Check sheet for the drawn part. Datum: minimum x, y, z corner. Units: mm. Round coordinates to 2 decimals unless told otherwise and drop trailing zeros. Write each loop counter-clockwise with the first axis right and the second up, starting at its lowest first coordinate (ties: lowest second). Pieces come first, ordered by that corner, then holes. Notation, with made-up numbers: M 64.25,-34 L 89.25,-34 A22 cw 89.25,-25 Z; hole C 45.25,4.25 d9. An arc over 180 degrees is marked long. One line per item, written item: value. Start each with the question number.
Item 1: Section check B-B, the plane y = 43. Record the cut outline in (x, z) (1 decimal), then the cut area to 3 significant figures.
Item 2: Section check D-D, the plane y = 35. Record the cut outline in (x, z), then the cut area to 3 significant figures.
Item 3: Gauge pin test, flat ends, axial feed: pin 1 (11 mm diameter, centred on x = 11, z = 38, fed in from -Y); pin 2 (6.5 mm diameter, centred on x = 17.5, z = 45, fed in from +Y); pin 3 (4 mm diameter, centred on x = 5, z = 61, fed in from -Y). Record the tip position at first contact, or that the pin passes through.
Item 4: Draft check along X on the marked faces 1, 2, 3 and 4. Enter one of: +X half, -X half, draft (parallel to the pull), parting line (faces both ways), or undercut.
Item 5: Thickness scan on probe 1 along X at (y, z) = (22.5, 23.5); probe 2 along Z at (x, y) = (11.75, 27.25); probe 3 along Y at (x, z) = (6, 45). Record the ranges inside material, lowest first. Write a range as from..to.
Item 6: Section check A-A, the plane z = 39. Record the cut outline in (x, y), then the cut area to 3 significant figures.
Item 7: Section check C-C, the plane x = 15. State how many separate pieces and enclosed holes the cut face has, then the cut area to 4 significant figures.
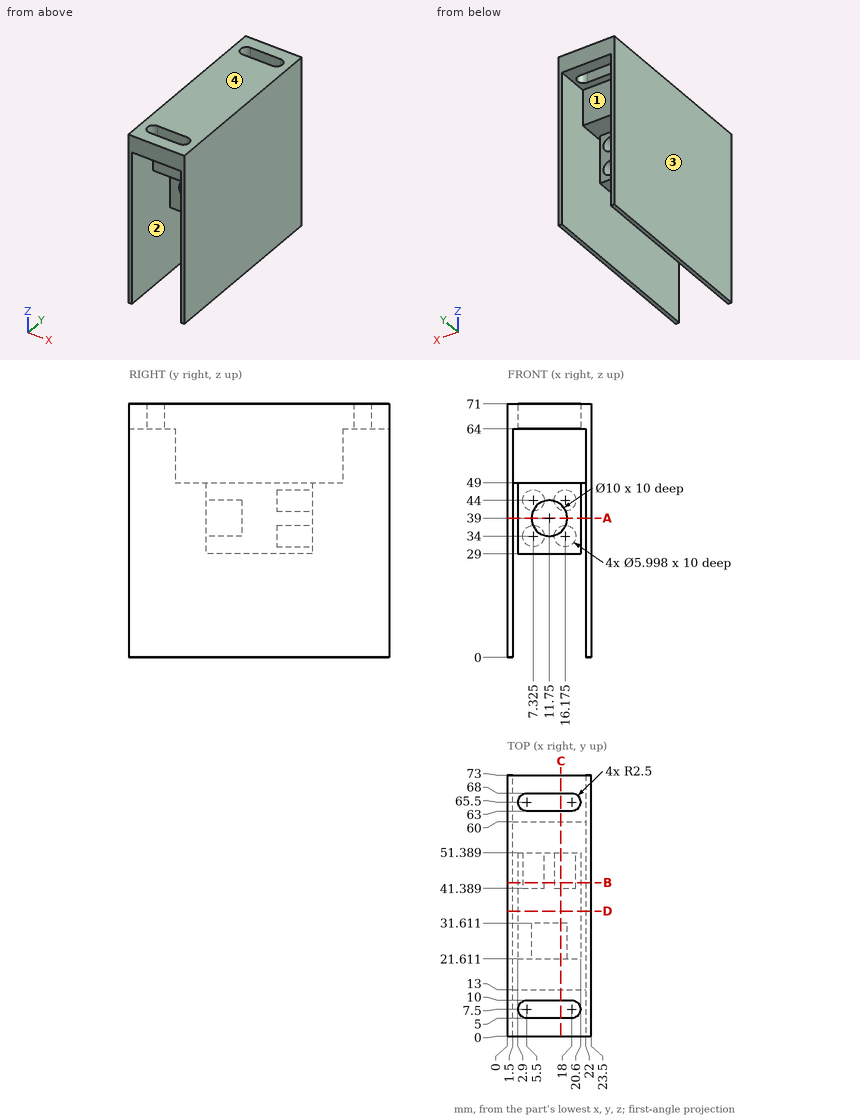
Response values:
1. outline: M 0,0 L 1.5,0 L 1.5,49 L 2.9,49 L 2.9,29 L 20.6,29 L 20.6,49 L 22,49 L 22,0 L 23.5,0 L 23.5,71 L 0,71 Z; hole C 7.3,34 d6; hole C 7.3,44 d6; hole C 16.2,34 d6; hole C 16.2,44 d6
1. area: 905 mm2
2. outline: M 0,0 L 1.5,0 L 1.5,49 L 2.9,49 L 2.9,29 L 20.6,29 L 20.6,49 L 22,49 L 22,0 L 23.5,0 L 23.5,71 L 0,71 Z
2. area: 1,020 mm2
3. pin 1: stops at y = 21.61
3. pin 2: stops at y = 51.39
3. pin 3: stops at y = 13
4. face 1: undercut
4. face 2: undercut
4. face 3: -X half
4. face 4: draft
5. probe 1: x = 0..1.5, 22..23.5
5. probe 2: z = 29..34, 44..71
5. probe 3: y = 21.61..41.39
6. outline: M 0,0 L 1.5,0 L 1.5,73 L 0,73 Z; M 2.9,21.61 L 6.75,21.61 L 6.75,31.61 L 16.75,31.61 L 16.75,21.61 L 20.6,21.61 L 20.6,51.39 L 2.9,51.39 Z; M 22,0 L 23.5,0 L 23.5,73 L 22,73 Z
6. area: 646 mm2
7. separate pieces: 3
7. enclosed holes: 0
7. area: 1,555 mm2
